```python
from build123d import *

# Parameters (mm, degrees)
SKETCH_1_R      = 2.475
EXTRUDE_1_DEPTH = 2
SKETCH_2_R      = 2.425
EXTRUDE_2_DEPTH = 3
SKETCH_3_R      = 2.45
EXTRUDE_3_DEPTH = 2
FILLET_1_R      = 0.2


with BuildPart() as part:
    # 스케치1 → 보스-돌출1 (new body)
    with BuildSketch(Plane.XY):
        Circle(SKETCH_1_R)
    extrude(amount=EXTRUDE_1_DEPTH)

    # 스케치2 → 보스-돌출2 (add)
    with BuildSketch(Plane.XY.offset(2)):
        Circle(SKETCH_2_R)
    extrude(amount=EXTRUDE_2_DEPTH)

    # 스케치3 → 보스-돌출3 (add)
    with BuildSketch(Plane.XY.offset(5)):
        Circle(SKETCH_3_R)
    extrude(amount=EXTRUDE_3_DEPTH)

    # 필렛1
    fillet_1_edges = [part.edges().sort_by_distance(p)[0] for p in [
        (-2.475, 0, 0),
        (-2.45, 0, 7),
    ]]
    fillet(fillet_1_edges, radius=FILLET_1_R)


solid = part.part
```
Design review of the part built by this model. Coordinates are the model's own, in mm. Round coordinates to 2 decimals unless told otherwise and drop trailing zeros. Order: outer loops, then holes, each group sorted by start corner. A loop starts at its lowest first (then second) coordinate and runs counter-clockwise, first axis right, second up. Notation, with made-up numbers: M -29,-23.5 L 17,-23.5 A19 cw 17,0.5 Z; hole C 19,-8.5 d6. An arc over 180 degrees is marked long. Put each result on its own line as item: value.
Q1. Consider section B-B (z = 5.75). State the section outline as (x, y) points, and give its area (3 significant figures).
Reported:
outline: C 0,0 d4.9
area: 18.9 mm²
Q2. Consider section A-A (z = 1.75). State the section outline as (x, y) points (3 decimals), and give its area (3 significant figures).
Reported:
outline: C 0,0 d4.95
area: 19.2 mm²
Q3. Draft analysis for pull direction Z (two halves, no side actions). For faces 1 (the face through (0, 0, 0)), 2 (the face through (2.313, 0.728, 3.479)), 3 (the face through (-0.5, -2.4, 5.9)), state which applies: released by +Z, released by -Z, zero draft, split by the parting line, or undercut.
Reported:
face 1: released by -Z
face 2: undercut
face 3: zero draft
Q4. Insertion check: pin 1 Ø2 at (x, z) = (-2, 3) entering from -Y; pin 2 Ø1.5 at (x, z) = (-1, 1.5) entering from +Y; pin 3 Ø2 at (x, z) = (1.5, 1.5) entering from -Y. Each pin has a flat end and moves straight along its axis. Give the tip position at first contact, or say it passes through.
Reported:
pin 1: y = -2.21
pin 2: y = 2.46
pin 3: y = -2.42
Q5. To check wall thickness, follow line 1 (X direction, y = 0.9, z = 3.5); line 2 (Z direction, x = -2.2, y = 0.6); line 3 (X direction, y = -1.85, z = 1.75). State the ranges of each line that lie inside material, in increasing order.
Reported:
line 1: -2.25 to 2.25
line 2: 0 to 7
line 3: -1.64 to 1.64
